Answer from the drawing. Dimensions are ordinates in mm from the lowest x, y and z of the part. Coordinates: 2 decimals unless noted, no trailing zeros. Write each loop counter-clockwise with the first axis right and the second up, starting at its lowest first coordinate (ties: lowest second). Pieces come first, ordered by that corner, then holes.
1) Each of these flat-tipped pins is pushed along its axis until it touches: pin 1 Ø3 at (x, z) = (1.5, 124) entering from +Y; pin 2 Ø1 at (x, z) = (3, 69) entering from -Y. Where does it stop, or does it pass through?
2) The part is cut by section C-C (y = 5.5). Determine the outline of the cut face in (x, z), then the cut area to 3 significant figures.
3) The part is cut by section B-B (x = 4.75). Determine the outline of the cut face in (y, z).
4) Find the intervals of material crossed by line 1 (X direction, y = 3.5, z = 162); line 2 (X direction, y = 1, z = 137.5), in increasing order.
5) The part is cut by section A-A (z = 78.5). Determine the outline of the cut face in (x, y).
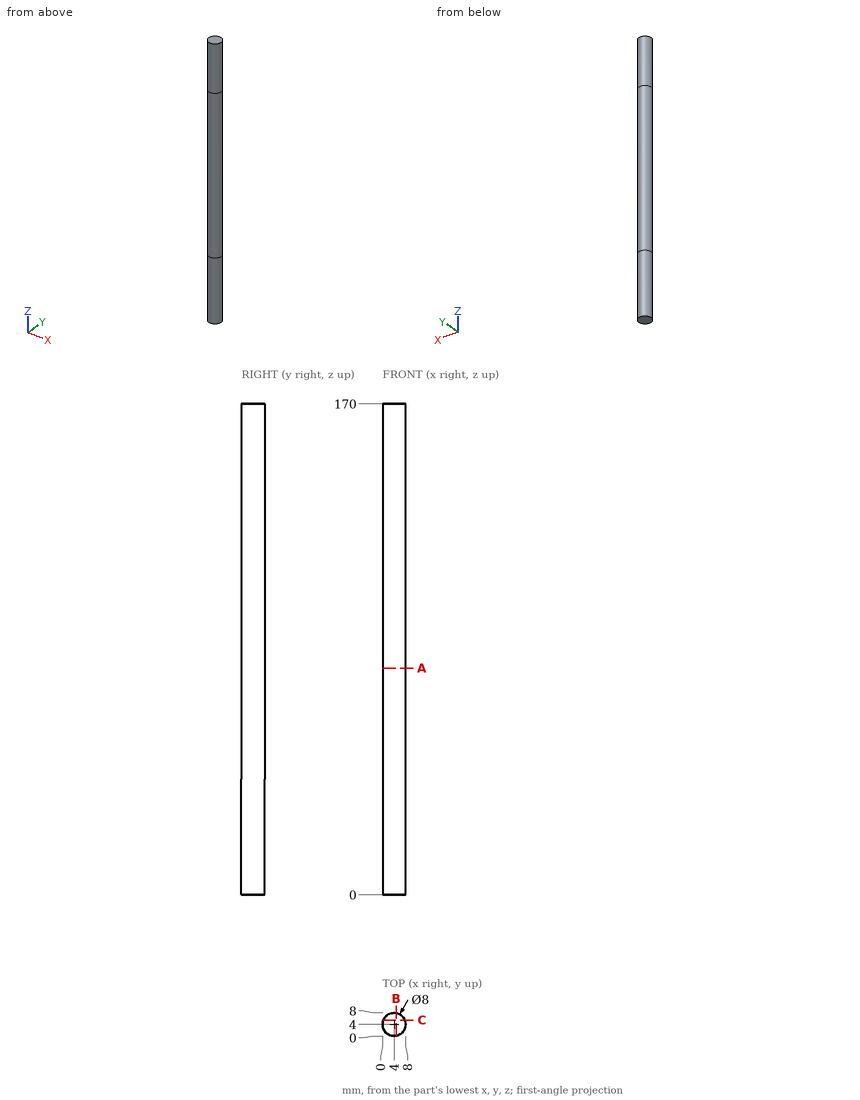
Reported:
1. pin 1: stops at y = 7.87
1. pin 2: stops at y = 0.03
2. outline: (0.29, 0) - (7.71, 0) - (7.71, 170) - (0.29, 170) - close
2. area: 1,260 mm2
3. outline: (0.07, 0) - (7.93, 0) - (7.93, 170) - (0.07, 170) - close
4. line 1: x = 0.03 to 7.97
4. line 2: x = 1.35 to 6.65
5. outline: circle Ø8 at (4, 4)
